Could you check a few things on this model? Use its own coordinates, in mm. A direction names the side the tool comes from. Round coordinates to 2 decimals unless told otherwise and drop trailing zeros. Write each loop counter-clockwise with the first axis right and the second up, starting at its lowest first coordinate (ties: lowest second). Pieces come first, ordered by that corner, then holes. Notation, with made-up numbers: (35, 41.25) - (75, 41.25) arc R23 cw to (75, 65.25) - close; hole circle Ø10 at (76.5, 34). An arc over 180 degrees is marked (long way). Write each question's results on one line, items separated by ' | '. Start each with the question number.
(1) Imagine slicing it at A-A on x = 28. Write out the boundary of the cut face in (y, z), then the cut area to 3 significant figures.
(2) Imagine slicing it at B-B on z = 18.5. Write out the boundary of the cut face in (x, y), then the cut area to 3 significant figures.
(3) For P1, Ø5, axis at y = 13, z = 33, coming from the +X side, with a flat end and sliding along its axis, tell me the tip position at first contact or that it passes through.
(4) On a 3-axis mill with a long thin cutter (end or side, diameter ignored), from which of +Z, -Z, +X, -X, +Y, -Y can I reach the whole of each face in a straight line? I mean faces 4 (the cylindrical face through (5.949, 22.345, 84.388)), 5 (the flat face through (3, 0, 0)). Say none if no direction works.
(5) Please list where these lines run through material, in increasing order: line 1 (Y direction, x = 17.5, z = 105.5); line 2 (X direction, y = 13.5, z = 52.5); line 3 (Y direction, x = 31, z = 19.5). Write a range as [from, to].
(6) Imagine slicing it at C-C on x = 17. Write out the boundary of the cut face in (y, z), then the cut area to 3 significant figures.
(7) Imagine slicing it at D-D on y = 7.5. Write out the boundary of the cut face in (x, z).
(8) Thinking about a two-plate mould opening in Y: for faces 1 (the cylindrical face through (6, -22.4, 84.4)), 2 (the flat face through (0, 0, 84)), 3 (the flat face through (18, 32.5, 84)), which applies, +Y half, -Y half, draft (parallel to the pull), parting line (faces both ways), or undercut?
Autodesk Inventor part; units mm, degrees
ref_plane "Начальная плоскость" through (0, 0, 0) normal (0, 0, 1) x (1, 0, 0)
ref_plane "Конечная плоскость" through (0, 0, 171.172) normal (0, 0, 1) x (1, 0, 0)
ref_plane "РабПлоскость8" through (169.3883, -32.5, 171.172) normal (0, 0, 1) x (1, 0, 0)
ref_plane "Начальная плоскость" through (0, 0, 0) normal (0, 0, 1) x (1, 0, 0)
ref_plane "Конечная плоскость" through (0, 0, 171.172) normal (0, 0, 1) x (1, 0, 0)
sketch "Эскиз" plane through (0, 0, 0) normal (0, 0, 1) x (1, 0, 0)
  line L0 (36, -32.5) -> (0, -32.5)
  line L1 (36, -32.5) -> (36, -28.696)
  line L2 (33.6994, -26.2039) -> (9.9215, -24.3017)
  line L3 (4.4, -18.3208) -> (4.4, 18.3208)
  line L4 (33.6994, 26.2039) -> (9.9215, 24.3017)
  line L5 (36, 28.696) -> (36, 32.5)
  line L6 (0, 32.5) -> (36, 32.5)
  line L7 (0, -32.5) -> (0, 32.5)
  arc A0 (4.4, -18.3208) -> (9.9215, -24.3017) centre (10.4, -18.3208) ccw
  arc A1 (9.9215, 24.3017) -> (4.4, 18.3208) centre (10.4, 18.3208) ccw
  arc A2 (36, -28.696) -> (33.6994, -26.2039) centre (33.5, -28.696) ccw
  arc A3 (33.6994, 26.2039) -> (36, 28.696) centre (33.5, 28.696) ccw
  line L8 (0, 45.5) -> (0, -45.5) construction
  line L9 (-7.2974, 0) -> (43.7847, 0) construction
  point P0 (36, -26.388)
  point P1 (4.4, -23.86)
  point P2 (4.4, 23.86)
  point P3 (36, 26.388)
  dimension "d3" = 36
  dimension "d5" = 4.4
  dimension "d7" = 65
  dimension "d9" = 8.64
  dimension "d11" = 8.64
  dimension "d13" = 6.112
  dimension "d15" = 6.112
  dimension "d22" = 6
  dimension "d23" = 2.5
  dimension "d24" = 32.5
  dimension "d25" = 0
extrude "Тело" add sketch "Эскиз" along normal up to surface (171.172 mm away) from surface at 0
sketch "Sketch3" plane through (0, 0, 0) normal (0, 0, 1) x (1, 0, 0)
  line L0 (0, 0) -> (10, 0)
ref_plane "Work Plane7" through (0, 0, 0) normal (0, -1, 0) x (1, 0, 0)
sketch "Sketch4" plane through (0, 0, 0) normal (0, -1, 0) x (1, 0, 0)
  line L0 (-2, 0) -> (12, 0)
  line L1 (-2, 171.172) -> (12, 171.172)
  dimension "d29" = 171.172
ref_plane "РабПлоскость8" through (169.3883, -32.5, 171.172) normal (0, 0, 1) x (1, 0, 0)
split "Разделение1" plane through (169.3883, -32.5, 171.172) removes the side toward (0, 0, 1)
equation "\"d3\" = b"
equation "\"d7\" = ParH"
equation "\"d22\" = R"
equation "\"d23\" = R1"
equation "\"d24\" = 0.5 * d7"
equation "\"d16\" = G_L"
equation "\"R1\" = 2.5"
equation "\"R\" = 6"
equation "\"t1\" = 4.4"
equation "\"t2\" = 7.2"
equation "\"ParH\" = 65"
equation "\"b\" = 36"
equation "\"msp_x1\" = 0.04 * b"
equation "\"msp_x2\" = -0.08 * t1 + 0.04 * b"
equation "\"G_L\" = d29"
equation "\"ex\" = 0"
equation "\"G_OFFSET_START\" = 0"
equation "\"G_OFFSET_END\" = -36"
equation "\"d27\" = G_OFFSET_END + B_L"
equation "\"B_L\" = 207.172"
properties part number "Швеллер 6.5U-171,17 ГОСТ 8240-97" material "Сталь, мягкая"
Response:
1) outline: (-32.5, 0) - (-25.75, 0) - (-25.75, 171.17) - (-32.5, 171.17) - close; (25.75, 0) - (32.5, 0) - (32.5, 171.17) - (25.75, 171.17) - close | area: 2,310 mm²
2) outline: (0, -32.5) - (36, -32.5) - (36, -28.7) arc R2.5 ccw to (33.7, -26.2) - (9.92, -24.3) arc R6 cw to (4.4, -18.32) - (4.4, 18.32) arc R6 cw to (9.92, 24.3) - (33.7, 26.2) arc R2.5 ccw to (36, 28.7) - (36, 32.5) - (0, 32.5) - close | area: 763 mm²
3) P1: x = 4.4
4) face 4: +Z, -Z, +X | face 5: -Z, +X, -X, +Y, -Y
5) line 1: [-32.5, -24.91], [24.91, 32.5] | line 2: [0, 4.4] | line 3: [-32.5, -25.99], [25.99, 32.5]
6) outline: (-32.5, 0) - (-24.87, 0) - (-24.87, 171.17) - (-32.5, 171.17) - close; (24.87, 0) - (32.5, 0) - (32.5, 171.17) - (24.87, 171.17) - close | area: 2,610 mm²
7) outline: (0, 0) - (4.4, 0) - (4.4, 171.17) - (0, 171.17) - close
8) face 1: undercut | face 2: draft | face 3: +Y half
